from build123d import *

# Parameters (mm, degrees)
ESQUISSE1_R          = 3.025
ESQUISSE1_R_2        = 0.85
BOSS_EXTRU_1_DEPTH   = 0.75
CONG_1_R             = 5
CONG_2_R             = 1
CHANFREIN1_START     = -11.517439791
CHANFREIN1_OUTLINE_W = 6
CHANFREIN1_OUTLINE_H = 4
CHANFREIN1_DEPTH     = 2.517439791
CONG_3_R             = 1
BOSS_EXTRU_2_DEPTH   = 1.5


with BuildPart() as part:
    # Esquisse1 → Boss.-Extru.1 (new, symmetric)
    with BuildSketch(Plane.XY):
        with BuildLine():
            Line((-21.5, 11), (1.242174044, 6.914306086))
            ThreePointArc((1.242174044, 6.914306086), (4.121125954, -5.689195538), (-6.957010852, 0.975))
            Line((-6.957010852, 0.975), (-21.5, 0.975))
            Line((-21.5, 0.975), (-21.5, -5))
            Line((-21.5, -5), (-35.5, -5))
            Line((-35.5, -5), (-35.5, 11))
            Line((-35.5, 11), (-21.5, 11))
        make_face()
        Circle(ESQUISSE1_R, mode=Mode.SUBTRACT)
        with Locations((-32.5, 8)):
            Circle(ESQUISSE1_R_2, mode=Mode.SUBTRACT)
        with Locations((-24.5, 8)):
            Circle(ESQUISSE1_R_2, mode=Mode.SUBTRACT)
        with Locations((-24.5, -2)):
            Circle(ESQUISSE1_R_2, mode=Mode.SUBTRACT)
        with Locations((-32.5, -2)):
            Circle(ESQUISSE1_R_2, mode=Mode.SUBTRACT)
    extrude(amount=BOSS_EXTRU_1_DEPTH, both=True)

    # Congé1
    cong_1_edges = [part.edges().sort_by_distance(p)[0] for p in [
        (-21.5, 11, 0),
        (-6.957010852, 0.975, 0),
        (-21.5, 0.975, 0),
    ]]
    fillet(cong_1_edges, radius=CONG_1_R)

    # Congé2
    cong_2_edges = [part.edges().sort_by_distance(p)[0] for p in [
        (-35.5, 11, 0),
        (-35.5, -5, 0),
    ]]
    fillet(cong_2_edges, radius=CONG_2_R)

    # Chanfrein1: read off the stored shape, not the designer's step
    # Chanfrein1 outline → Chanfrein1 (cut)
    with BuildSketch(Plane(origin=(0, 0, 0), x_dir=(0.7571091636707948, 0.6532883852371091, 0), z_dir=(0.6532883852371091, -0.7571091636707951, 0)).offset(CHANFREIN1_START)):
        with Locations((-20, 0)):
            Rectangle(CHANFREIN1_OUTLINE_W, CHANFREIN1_OUTLINE_H)
    extrude(amount=CHANFREIN1_DEPTH, mode=Mode.SUBTRACT)

    # Congé3
    cong_3_edges = [part.edges().sort_by_distance(p)[0] for p in [
        (-21.44610623, -3.292857143, 0),
        (-23.424548722, -5, 0),
    ]]
    fillet(cong_3_edges, radius=CONG_3_R)

    # Esquisse2 → Boss.-Extru.2 (add)
    with BuildSketch(Plane.XY.offset(0.75)):
        with BuildLine():
            Line((-21.945565237, 11), (2.464036076, 6.578689171))
            ThreePointArc((2.464036076, 6.578689171), (-9.542172297, 9.885752111), (-21.945565237, 11))
        make_face()
    extrude(amount=-BOSS_EXTRU_2_DEPTH)


solid = part.part
Geometry check sheet. Reference: the model listing, model coordinates, mm. A direction names the side the tool comes from. Coordinates: 2 decimals unless noted, no trailing zeros. Write each loop counter-clockwise with the first axis right and the second up, starting at its lowest first coordinate (ties: lowest second). Pieces come first, ordered by that corner, then holes. Notation, with made-up numbers: (17.5, -1) -> (63.5, -1) arc R27 ccw to (63.5, 20) -> close; hole circle Ø5 at (-1, 68). An arc over 180 degrees is marked (long way). One line per question, with ' | ' between items.
1. Cross-section at A-A on x = -32.5. Record the cut outline in (y, z), and give its area (3 significant figures).
Answers:
outline: (-5, -0.75) -> (-2.85, -0.75) -> (-2.85, 0.75) -> (-5, 0.75) -> close; (-1.15, -0.75) -> (7.15, -0.75) -> (7.15, 0.75) -> (-1.15, 0.75) -> close; (8.85, -0.75) -> (11, -0.75) -> (11, 0.75) -> (8.85, 0.75) -> close | area: 18.9 mm²
2. Cross-section at B-B on z = -0.5. Record the cut outline in (x, y) (3 decimals), and give its area (3 significant figures).
Answers:
outline: (-35.5, -4) arc R1 ccw to (-34.5, -5) -> (-23.796, -5) arc R1 ccw to (-23.143, -4.757) -> (-21.713, -3.523) arc R1 ccw to (-21.389, -2.976) arc R5 cw to (-16.5, 0.975) -> (-11.331, 0.975) arc R5 cw to (-6.62, -2.351) arc R7.025 ccw (long way) to (2.464, 6.579) arc R69.592 ccw to (-21.946, 11) -> (-34.5, 11) arc R1 ccw to (-35.5, 10) -> close; hole circle Ø1.7 at (-32.5, -2); hole circle Ø1.7 at (-32.5, 8); hole circle Ø1.7 at (-24.5, -2); hole circle Ø1.7 at (-24.5, 8); hole circle Ø6.05 at (0, 0) | area: 506 mm²
3. Set-up check for faces 1 (the cylindrical face through (-8.48, 0.08, -0.01)), 2 (the cylindrical face through (-33.35, -1.96, -0.01)), 3 (the flat face through (-29, -5, 0)): record each of +Z, -Z, +X, -X, +Y, -Y from which the full face is reachable in a straight line by a thin tool's end or side.
Answers:
face 1: +Z, -Z, -Y | face 2: +Z, -Z | face 3: +Z, -Z, -X, -Y
4. Thickness scan on probe 1 along Y at (x, z) = (-24.5, 0.4); probe 2 along X at (y, z) = (-1.5, 0.4); probe 3 along X at (y, z) = (-0.5, 0.55). Record the ranges inside material, lowest first. Write a range as from..to.
Answers:
probe 1: y = -5..-2.85, -1.15..7.15, 8.85..11 | probe 2: x = -35.5..-33.19, -31.81..-25.19, -23.81..-20.82, -7.02..-2.63, 2.63..6.86 | probe 3: x = -35.5..-20.05, -7.79..-2.98, 2.98..7.01
5. Cross-section at D-D on x = 2. Record the cut outline in (y, z).
Answers:
outline: (-6.73, -0.75) -> (-2.27, -0.75) -> (-2.27, 0.75) -> (-6.73, 0.75) -> close; (2.27, -0.75) -> (6.75, -0.75) -> (6.75, 0.75) -> (2.27, 0.75) -> close
6. Cross-section at C-C on y = 1.75. Record the cut outline in (x, z).
Answers:
outline: (-35.5, -0.75) -> (-2.47, -0.75) -> (-2.47, 0.75) -> (-35.5, 0.75) -> close; (2.47, -0.75) -> (6.8, -0.75) -> (6.8, 0.75) -> (2.47, 0.75) -> close
